Read the model definition and answer for the solid it produces. Units are mm, in the model's axes. Face numbers are marked on the shaded views. A direction names the side the tool comes from. Give positions to 0.01 mm unless a question says otherwise; leave off trailing zeros. Order: outer loops, then holes, each group sorted by start corner. A loop starts at its lowest first (then second) coordinate and runs counter-clockwise, first axis right, second up. Notation, with made-up numbers: (74, 63.5) - (80, 63.5) arc R23 cw to (80, 87.5) - close; hole circle Ø5 at (85, -7.75). An arc over 180 degrees is marked (long way). Write each question's results on one line, items separated by ' | '.
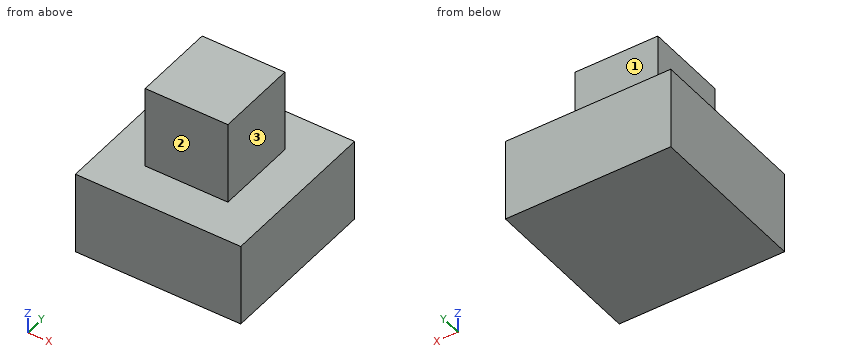
from build123d import *

# Parameters (mm, degrees)
SKETCH_1_W                = 20
SKETCH_1_H                = 20
BASEBOX_DEPTH             = 10
SKETCH_2_W                = 10
SKETCH_2_H                = 10
DRAFTDIR2_DEPTH           = 10
DRAFTDIR2_OTHER_WAY_DEPTH = 5
DRAFTDIR2_OTHER_WAY_TAPER = 3


with BuildPart() as part:
    # 草图1 → BaseBox (new body)
    with BuildSketch(Plane.XY):
        with Locations((10, 10)):
            Rectangle(SKETCH_1_W, SKETCH_1_H)
    extrude(amount=BASEBOX_DEPTH)

    # 草图2 → DraftDir2 (add)
    with BuildSketch(Plane.XY.offset(10)):
        with Locations((10, 10)):
            Rectangle(SKETCH_2_W, SKETCH_2_H)
    extrude(amount=DRAFTDIR2_DEPTH)

    # 草图2 → DraftDir2 other way (add)
    with BuildSketch(Plane.XY.offset(10)):
        with Locations((10, 10)):
            Rectangle(SKETCH_2_W, SKETCH_2_H)
    extrude(amount=-DRAFTDIR2_OTHER_WAY_DEPTH, taper=DRAFTDIR2_OTHER_WAY_TAPER)


solid = part.part
(1) Section C-C (z = 16.5) is taken. Give the vertices of the cut face in (x, y), plus the area to 3 significant figures.
Conclusion:
outline: (5, 5) - (15, 5) - (15, 15) - (5, 15) - close | area: 100 mm^2
(2) Section D-D (y = 1.5) is taken. Give the vertices of the cut face in (x, z).
Conclusion:
outline: (0, 0) - (20, 0) - (20, 10) - (0, 10) - close
(3) Consider probe 1 along Z at (x, y) = (4, 10); probe 2 along Y at (x, z) = (8, 15). Determine where each line is inside the solid, lowest interval first. Write a range as [from, to].
Conclusion:
probe 1: [0, 10] | probe 2: [5, 15]
(4) Each of these flat-tipped pins is pushed along its axis until it touches: pin 1 (12 mm diameter, centred on x = 5.5, z = 18, fed in from +Y); pin 2 (1 mm diameter, centred on x = 16.5, z = 16.5, fed in from -Y); pin 3 (3 mm diameter, centred on y = 8, z = 12.5, fed in from -X); pin 4 (3 mm diameter, centred on x = 13.5, z = 17.5, fed in from -Y). Where does it stop, or does it pass through?
Conclusion:
pin 1: y = 15 | pin 2: through | pin 3: x = 5 | pin 4: y = 5
(5) Section A-A (y = 7.75) is taken. Give the vertices of the cut face in (x, z).
Conclusion:
outline: (0, 0) - (20, 0) - (20, 10) - (15, 10) - (15, 20) - (5, 20) - (5, 10) - (0, 10) - close
(6) For the marked faces 1, 2 and 3, determine the directions among +Z, -Z, +X, -X, +Y, -Y from which every point of the face is accessible in a straight line to the end or side of a thin tool.
Conclusion:
face 1: +Z, +X, -X, +Y | face 2: +Z, +X, -X, -Y | face 3: +Z, +X, +Y, -Y
